Geometry check sheet. Reference: the model listing, model coordinates, mm. A direction names the side the tool comes from. Coordinates: 2 decimals unless noted, no trailing zeros. Write each loop counter-clockwise with the first axis right and the second up, starting at its lowest first coordinate (ties: lowest second). Pieces come first, ordered by that corner, then holes. Notation, with made-up numbers: M 34.5,31 L 47.5,31 A32 cw 47.5,70 Z; hole C 33.5,-35.75 d9. An arc over 180 degrees is marked long. Put each result on its own line as item: value. Start each with the question number.
1) Cross-section at B-B on x = 8.5. Record the cut outline in (y, z).
2) Mould release check, pull along X, two halves, no side actions. Record for faces 3 (the flat face through (19.586, 18, 1)), 4 (the flat face through (22, 14, 3)), 5 (the flat face through (0.886, 18, 1)), 6 (the cylindrical face through (13.763, 37.806, 1.479)): released by +X, released by -X, zero draft, split by the parting line, or undercut.
3) Set-up check for faces 1 (the flat face through (14, 6.709, 1)), 2 (the cylindrical face through (13.209, -1.388, 1.479)): record each of +Z, -Z, +X, -X, +Y, -Y from which the full face is reachable in a straight line by a thin tool's end or side.
4) Cross-section at C-C on z = 2.15. Record the cut outline in (x, y), plus the area to 3 significant figures.
5) Cross-section at D-D on y = 3.5. Record the cut outline in (x, z), plus the area to 3 significant figures.
6) Gauge pin test, flat ends, axial feed: pin 1 (1.5 mm diameter, centred on x = 12.5, z = 1, fed in from -Y); pin 2 (1.8 mm diameter, centred on x = 22.59, y = 18.21, fed in from -Z); pin 3 (1.6 mm diameter, centred on y = 30.5, z = 1.5, fed in from +X); pin 4 (1.5 mm diameter, centred on y = 32, z = 0.5, fed in from +X). Record the tip position at first contact, or that the pin passes through.
7) Cross-section at A-A on y = 15. Record the cut outline in (x, z).
8) Scan lines: line 1 along X through (y, z) = (25.5, 2.5); line 2 along Y through (x, z) = (22.75, 0.15); line 3 along Y through (x, z) = (11, 0.3). Record each from-to range of solid material in increasing order.
from build123d import *

# Parameters (mm, degrees)
MODEL_R             = 1.5
BOSS_EXTRUDE1_DEPTH = 3


with BuildPart() as part:
    # Model → Boss-Extrude1 (new body)
    with BuildSketch(Plane.XY):
        with BuildLine():
            Line((0.88624, 25.209089561), (0.88624, 11.208991882))
            ThreePointArc((0.88624, 11.208991882), (13.486238839, -1.391009279), (26.08624, 11.20898956))
            Line((26.08624, 11.20898956), (26.08624, 16.208989561))
            Line((26.08624, 16.208989561), (26.08624, 25.208989561))
            ThreePointArc((26.08624, 25.208989561), (13.48629, 37.809039561), (0.88624, 25.209089561))
        make_face()
        with Locations((4.586289997, 18.209039557)):
            Circle(MODEL_R, mode=Mode.SUBTRACT)
        with Locations((22.586289997, 18.209039557)):
            Circle(MODEL_R, mode=Mode.SUBTRACT)
        Polygon((19.58624, 6.708989561), (19.58624, 29.708989561), (16.08624, 29.708989561), (16.08624, 31.708989561), (11.08624, 31.708989561), (11.08624, 29.708989561), (7.58624, 29.708989561), (7.58624, 6.708989561), align=None, mode=Mode.SUBTRACT)
    extrude(amount=BOSS_EXTRUDE1_DEPTH)


solid = part.part
Answer key:
1. outline: M -0.36,0 L 6.71,0 L 6.71,3 L -0.36,3 Z; M 29.71,0 L 36.78,0 L 36.78,3 L 29.71,3 Z
2. face 3: undercut
2. face 4: zero draft
2. face 5: released by -X
2. face 6: split by the parting line
3. face 1: +Z, -Z
3. face 2: +Z, -Z, -Y
4. outline: M 0.89,11.21 A12.6 ccw 26.09,11.21 L 26.09,25.21 A12.6 ccw 0.89,25.21 Z; hole C 4.59,18.21 d3; hole M 7.59,6.71 L 19.59,6.71 L 19.59,29.71 L 16.09,29.71 L 16.09,31.71 L 11.09,31.71 L 11.09,29.71 L 7.59,29.71 Z; hole C 22.59,18.21 d3
4. area: 551 mm²
5. outline: M 3.52,0 L 23.45,0 L 23.45,3 L 3.52,3 Z
5. area: 59.8 mm²
6. pin 1: stops at y = -1.39
6. pin 2: passes through
6. pin 3: stops at x = 25.26
6. pin 4: stops at x = 24.54
7. outline: M 0.89,0 L 7.59,0 L 7.59,3 L 0.89,3 Z; M 19.59,0 L 26.09,0 L 26.09,3 L 19.59,3 Z
8. line 1: x = 0.89 to 7.59, 19.59 to 26.08
8. line 2: y = 2.67 to 16.72, 19.7 to 33.75
8. line 3: y = -1.14 to 6.71, 29.71 to 37.56
